Check sheet for the modelled part. Datum: model origin and axes. Units: mm. A direction names the side the tool comes from. Round coordinates to 2 decimals unless told otherwise and drop trailing zeros. Loops run counter-clockwise (first coordinate to the right, second up) from the corner with the lowest first, then second, coordinate; pieces in that order, holes last. Notation, with made-up numbers: (-25.5, 71) - (-16.5, 71) arc R28 ccw to (-16.5, 108) - close; hole circle Ø1 at (86.25, 89.25). An arc over 180 degrees is marked (long way). Answer in a Markdown table with one row per item. Add a question column.
(1) Gauge pin test, flat end, axial feed: pin 1 (4 mm diameter, centred on x = 0, z = 0, fed in from -Y). Record the tip position at first contact, or that the pin passes through.
(2) Thickness scan on line 1 along Z through (x, y) = (0, -0.3); line 2 along X through (y, z) = (-0.9, 4); line 3 along X through (y, z) = (-0.35, -3.75). Record the ranges inside material, lowest first.
(3) Mould release check, pull along Z, two halves, no side actions. Record for faces 1 (the flat face through (-0.904, -0.626, 4.121)), 2 (the flat face through (-1.4, 0, 1.4)), 3 (the flat face through (3.63, -0.63, -2.13)), 4 (the cylindrical face through (-0.385, -0.626, -1.736)): +Z half, -Z half, draft (parallel to the pull), parting line (faces both ways), or undercut.
(4) Cross-section at A-A on z = 2.75. Enter the section's corners in (x, y), then the cut area to 3 significant figures.
(5) Access from +Z, -Z, +X, -X, +Y, -Y to the whole of each face (thin tool, end or side, straight path). Record for faces 5 (the flat face through (0.906, -0.626, 4.109)), 6 (the flat face through (-1.4, -1.27, 1.4)), 7 (the flat face through (-0.906, -0.626, -4.109)), 8 (the flat face through (-3.63, -0.63, 2.13)).
(6) Cross-section at B-B on z = 5.25. Enter the section's corners in (x, y), then the cut area to 3 significant figures.
from build123d import *

# Parameters (mm, degrees)
F0_R     = 3.556
F1_DEPTH = 2.54
F2_R     = 5.08
F3_R     = 1.016
F4_SCALE = 0.5


with BuildPart() as f1:
    # F0 (on Front) → F1 (new body)
    with BuildSketch(Plane.XZ):
        with BuildLine():
            ThreePointArc((7.6056039975, -0.4681750033), (7.616400149, -0.2341981419), (7.62, 0))
            ThreePointArc((7.62, 0), (7.616400149, 0.2341981419), (7.6056039975, 0.4681750033))
            ThreePointArc((7.6056039975, 0.4681750033), (7.2470506542, 2.3547094971), (6.4282492489, 4.0917003304))
            ThreePointArc((6.4282492489, 4.0917003304), (6.1647094971, 4.4789236225), (5.877876524, 4.8492233985))
            ThreePointArc((5.877876524, 4.8492233985), (4.4789236225, 6.1647094971), (2.7955217754, 7.0886852098))
            ThreePointArc((2.7955217754, 7.0886852098), (2.3547094971, 7.2470506542), (1.905, 7.3780332745))
            ThreePointArc((1.905, 7.3780332745), (0, 7.62), (-1.905, 7.3780332745))
            ThreePointArc((-1.905, 7.3780332745), (-2.3547094971, 7.2470506542), (-2.7955217754, 7.0886852098))
            ThreePointArc((-2.7955217754, 7.0886852098), (-4.4789236225, 6.1647094971), (-5.877876524, 4.8492233985))
            ThreePointArc((-5.877876524, 4.8492233985), (-6.1647094971, 4.4789236225), (-6.4282492489, 4.0917003304))
            ThreePointArc((-6.4282492489, 4.0917003304), (-7.2470506542, 2.3547094971), (-7.6056039975, 0.4681750033))
            ThreePointArc((-7.6056039975, 0.4681750033), (-7.62, 0), (-7.6056039975, -0.4681750033))
            ThreePointArc((-7.6056039975, -0.4681750033), (-7.2470506542, -2.3547094971), (-6.4282492489, -4.0917003304))
            ThreePointArc((-6.4282492489, -4.0917003304), (-6.1647094971, -4.4789236225), (-5.877876524, -4.8492233985))
            ThreePointArc((-5.877876524, -4.8492233985), (-4.4789236225, -6.1647094971), (-2.7955217754, -7.0886852098))
            ThreePointArc((-2.7955217754, -7.0886852098), (-2.3547094971, -7.2470506542), (-1.905, -7.3780332745))
            ThreePointArc((-1.905, -7.3780332745), (0, -7.62), (1.905, -7.3780332745))
            ThreePointArc((1.905, -7.3780332745), (2.3547094971, -7.2470506542), (2.7955217754, -7.0886852098))
            ThreePointArc((2.7955217754, -7.0886852098), (4.4789236225, -6.1647094971), (5.877876524, -4.8492233985))
            ThreePointArc((5.877876524, -4.8492233985), (6.1647094971, -4.4789236225), (6.4282492489, -4.0917003304))
            ThreePointArc((6.4282492489, -4.0917003304), (7.2470506542, -2.3547094971), (7.6056039975, -0.4681750033))
        make_face()
        Circle(F0_R, mode=Mode.SUBTRACT)
        with BuildLine():
            ThreePointArc((6.4282492489, 4.0917003304), (7.2470506542, 2.3547094971), (7.6056039975, 0.4681750033))
            Line((7.6056039975, 0.4681750033), (9.689784553, 1.4124377213))
            Line((9.689784553, 1.4124377213), (11.8307519964, 3.04283013))
            Line((11.8307519964, 3.04283013), (11.359810097, 4.4922402608))
            Line((11.359810097, 4.4922402608), (8.6694104376, 4.5528263381))
            Line((8.6694104376, 4.5528263381), (6.4282492489, 4.0917003304))
        make_face()
        with BuildLine():
            Line((9.689784553, -1.4124377213), (7.6056039975, -0.4681750033))
            ThreePointArc((7.6056039975, -0.4681750033), (7.2470506542, -2.3547094971), (6.4282492489, -4.0917003304))
            Line((6.4282492489, -4.0917003304), (8.6694104376, -4.5528263381))
            Line((8.6694104376, -4.5528263381), (11.359810097, -4.4922402608))
            Line((11.359810097, -4.4922402608), (11.8307519964, -3.04283013))
            Line((11.8307519964, -3.04283013), (9.689784553, -1.4124377213))
        make_face()
        with BuildLine():
            ThreePointArc((2.7955217754, 7.0886852098), (4.4789236225, 6.1647094971), (5.877876524, 4.8492233985))
            Line((5.877876524, 4.8492233985), (7.0089903128, 6.8381985782))
            Line((7.0089903128, 6.8381985782), (7.7827487457, 9.4156428332))
            Line((7.7827487457, 9.4156428332), (6.5498068462, 10.3114275577))
            Line((6.5498068462, 10.3114275577), (4.3376161974, 8.7790654812))
            Line((4.3376161974, 8.7790654812), (2.7955217754, 7.0886852098))
        make_face()
        with BuildLine():
            Line((7.0089903128, -6.8381985782), (5.877876524, -4.8492233985))
            ThreePointArc((5.877876524, -4.8492233985), (4.4789236225, -6.1647094971), (2.7955217754, -7.0886852098))
            Line((2.7955217754, -7.0886852098), (4.3376161974, -8.7790654812))
            Line((4.3376161974, -8.7790654812), (6.5498068462, -10.3114275577))
            Line((6.5498068462, -10.3114275577), (7.7827487457, -9.4156428332))
            Line((7.7827487457, -9.4156428332), (7.0089903128, -6.8381985782))
        make_face()
        with BuildLine():
            ThreePointArc((-1.905, 7.3780332745), (0, 7.62), (1.905, 7.3780332745))
            Line((1.905, 7.3780332745), (1.651, 9.652))
            Line((1.651, 9.652), (0.762, 12.192))
            Line((0.762, 12.192), (-0.762, 12.192))
            Line((-0.762, 12.192), (-1.651, 9.652))
            Line((-1.651, 9.652), (-1.905, 7.3780332745))
        make_face()
        with BuildLine():
            Line((1.651, -9.652), (1.905, -7.3780332745))
            ThreePointArc((1.905, -7.3780332745), (0, -7.62), (-1.905, -7.3780332745))
            Line((-1.905, -7.3780332745), (-1.651, -9.652))
            Line((-1.651, -9.652), (-0.762, -12.192))
            Line((-0.762, -12.192), (0.762, -12.192))
            Line((0.762, -12.192), (1.651, -9.652))
        make_face()
        with BuildLine():
            ThreePointArc((-5.877876524, 4.8492233985), (-4.4789236225, 6.1647094971), (-2.7955217754, 7.0886852098))
            Line((-2.7955217754, 7.0886852098), (-4.3376161974, 8.7790654812))
            Line((-4.3376161974, 8.7790654812), (-6.5498068462, 10.3114275577))
            Line((-6.5498068462, 10.3114275577), (-7.7827487457, 9.4156428332))
            Line((-7.7827487457, 9.4156428332), (-7.0089903128, 6.8381985782))
            Line((-7.0089903128, 6.8381985782), (-5.877876524, 4.8492233985))
        make_face()
        with BuildLine():
            Line((-4.3376161974, -8.7790654812), (-2.7955217754, -7.0886852098))
            ThreePointArc((-2.7955217754, -7.0886852098), (-4.4789236225, -6.1647094971), (-5.877876524, -4.8492233985))
            Line((-5.877876524, -4.8492233985), (-7.0089903128, -6.8381985782))
            Line((-7.0089903128, -6.8381985782), (-7.7827487457, -9.4156428332))
            Line((-7.7827487457, -9.4156428332), (-6.5498068462, -10.3114275577))
            Line((-6.5498068462, -10.3114275577), (-4.3376161974, -8.7790654812))
        make_face()
        with BuildLine():
            ThreePointArc((-7.6056039975, 0.4681750033), (-7.2470506542, 2.3547094971), (-6.4282492489, 4.0917003304))
            Line((-6.4282492489, 4.0917003304), (-8.6694104376, 4.5528263381))
            Line((-8.6694104376, 4.5528263381), (-11.359810097, 4.4922402608))
            Line((-11.359810097, 4.4922402608), (-11.8307519964, 3.04283013))
            Line((-11.8307519964, 3.04283013), (-9.689784553, 1.4124377213))
            Line((-9.689784553, 1.4124377213), (-7.6056039975, 0.4681750033))
        make_face()
        with BuildLine():
            Line((-8.6694104376, -4.5528263381), (-6.4282492489, -4.0917003304))
            ThreePointArc((-6.4282492489, -4.0917003304), (-7.2470506542, -2.3547094971), (-7.6056039975, -0.4681750033))
            Line((-7.6056039975, -0.4681750033), (-9.689784553, -1.4124377213))
            Line((-9.689784553, -1.4124377213), (-11.8307519964, -3.04283013))
            Line((-11.8307519964, -3.04283013), (-11.359810097, -4.4922402608))
            Line((-11.359810097, -4.4922402608), (-8.6694104376, -4.5528263381))
        make_face()
    extrude(amount=F1_DEPTH)

    # F2
    f2_edges = [f1.edges().sort_by_distance(p)[0] for p in [
        (7.00899, -1.27, 6.838199),
        (4.337616, -1.27, 8.779065),
        (1.651, -1.27, 9.652),
        (-4.337616, -1.27, 8.779065),
        (-8.66941, -1.27, 4.552826),
        (-9.689785, -1.27, -1.412438),
        (-7.00899, -1.27, -6.838199),
        (-1.651, -1.27, -9.652),
        (4.337616, -1.27, -8.779065),
        (8.66941, -1.27, -4.552826),
        (9.689785, -1.27, 1.412438),
        (9.689785, -1.27, -1.412438),
        (8.66941, -1.27, 4.552826),
        (-1.651, -1.27, 9.652),
        (-7.00899, -1.27, 6.838199),
        (-9.689785, -1.27, 1.412438),
        (-8.66941, -1.27, -4.552826),
        (-4.337616, -1.27, -8.779065),
        (1.651, -1.27, -9.652),
        (7.00899, -1.27, -6.838199),
    ]]
    fillet(f2_edges, radius=F2_R)

    # F3
    f3_edges = [f1.edges().sort_by_distance(p)[0] for p in [
        (0.762, -1.27, 12.192),
        (-0.762, -1.27, 12.192),
        (-6.549807, -1.27, 10.311428),
        (-7.782749, -1.27, 9.415643),
        (-11.35981, -1.27, 4.49224),
        (6.549807, -1.27, 10.311428),
        (7.782749, -1.27, 9.415643),
        (11.35981, -1.27, 4.49224),
        (-11.830752, -1.27, 3.04283),
        (-11.830752, -1.27, -3.04283),
        (-11.35981, -1.27, -4.49224),
        (-7.782749, -1.27, -9.415643),
        (-6.549807, -1.27, -10.311428),
        (-0.762, -1.27, -12.192),
        (0.762, -1.27, -12.192),
        (6.549807, -1.27, -10.311428),
        (7.782749, -1.27, -9.415643),
        (11.830752, -1.27, -3.04283),
        (11.35981, -1.27, -4.49224),
        (11.830752, -1.27, 3.04283),
    ]]
    fillet(f3_edges, radius=F3_R)


with BuildPart() as f1_1:
    # F4: moved
    add(f1.part.scale(F4_SCALE))


solid = f1_1.part
Answers:
| question | item | result |
|---|---|---|
| 1 | pin 1 | stops at y = -1.27 |
| 2 | line 1 | z = -6.1 to -1.78, 1.78 to 6.1 |
| 2 | line 2 | x = -3.68 to -1.81, -0.92 to 0.92, 1.81 to 3.68 |
| 2 | line 3 | x = -3.6 to -1.59, -0.95 to 0.95, 1.59 to 3.6 |
| 3 | face 1 | +Z half |
| 3 | face 2 | draft |
| 3 | face 3 | undercut |
| 3 | face 4 | undercut |
| 4 | outline | (-3.12, -1.27) - (3.12, -1.27) - (3.12, 0) - (-3.12, 0) - close |
| 4 | area | 7.93 mm^2 |
| 5 | face 5 | +Z, +Y, -Y |
| 5 | face 6 | +Z, -Z, +X, -X, -Y |
| 5 | face 7 | -Z, +Y, -Y |
| 5 | face 8 | +Y, -Y |
| 6 | outline | (-0.68, -1.27) - (0.68, -1.27) - (0.68, 0) - (-0.68, 0) - close |
| 6 | area | 1.72 mm^2 |
